from build123d import *

# Parameters (mm, degrees)
IZIM1_R                     = 3.5
IZIM1_R_2                   = 1.05
Y_KSEKLIK_EKSTR_ZYON1_DEPTH = 4
IZIM1_5_R                   = 0.5
Y_KSEKLIK_EKSTR_ZYON2_DEPTH = 1.8
IZIM2_R                     = 2.5
KES_EKSTR_ZYON1_DEPTH       = 2


with BuildPart() as part:
    # izim1 → Y_kseklik-Ekstr_zyon1 (new body)
    with BuildSketch(Plane(origin=(0, 0, 0), x_dir=(0, 0, -1), z_dir=(1, 0, 0))):
        with Locations((585.534826128, 415.055894204)):
            Circle(IZIM1_R)
        with Locations((585.534826128, 415.055894204)):
            Circle(IZIM1_R_2, mode=Mode.SUBTRACT)
    extrude(amount=Y_KSEKLIK_EKSTR_ZYON1_DEPTH)

    # izim1_5 → Y_kseklik-Ekstr_zyon2 (add)
    with BuildSketch(Plane(origin=(0, 0, 0), x_dir=(0, 0, -1), z_dir=(1, 0, 0))):
        with BuildLine():
            Line((583.367103568, 428.530198932), (582.052256525, 415.40476232))
            ThreePointArc((582.052256525, 415.40476232), (585.553599597, 418.555843854), (589.020937835, 415.367382833))
            Line((589.020937835, 415.367382833), (587.846970124, 428.506169262))
            ThreePointArc((587.846970124, 428.506169262), (585.617966971, 430.555894204), (583.367103568, 428.530198932))
        make_face()
        with Locations((585.566071769, 420.8810388)):
            Circle(IZIM1_5_R, mode=Mode.SUBTRACT)
        with Locations((585.57894519, 423.2810388)):
            Circle(IZIM1_5_R, mode=Mode.SUBTRACT)
        with Locations((585.591818611, 425.6810388)):
            Circle(IZIM1_5_R, mode=Mode.SUBTRACT)
        with Locations((585.604692031, 428.0810388)):
            Circle(IZIM1_5_R, mode=Mode.SUBTRACT)
    extrude(amount=Y_KSEKLIK_EKSTR_ZYON2_DEPTH)

    # izim2 → Kes-Ekstr_zyon1 (cut)
    with BuildSketch(Plane(origin=(4, 0, 0), x_dir=(0, 0, -1), z_dir=(1, 0, 0))):
        with Locations((585.534826128, 415.055894204)):
            Circle(IZIM2_R)
    extrude(amount=-KES_EKSTR_ZYON1_DEPTH, mode=Mode.SUBTRACT)


solid = part.part
Work out the finished part from the listing and answer in its coordinate system (mm). A direction names the side the tool comes from. Give positions to 0.01 mm unless a question says otherwise; leave off trailing zeros. Order: outer loops, then holes, each group sorted by start corner. A loop starts at its lowest first (then second) coordinate and runs counter-clockwise, first axis right, second up. Notation, with made-up numbers: (22.25, -25.75) - (66.25, -25.75) arc R23 ccw to (66.25, 7.25) - close; hole circle Ø3 at (26, 21). An arc over 180 degrees is marked (long way). Answer as CSV lines item,"result". Start each with the question number.
Q1. Find the intervals of material crossed by L1, parallel to Y at x = 2.6, z = -585.5; L2, parallel to X at y = 418.5, z = -584.25; L3, parallel to Z at x = 3.25, y = 417, in increasing order. Write a range as [from, to].
Q2. The part is cut by section D-D (x = 2.55). Write down the section's boundary in (y, z).
Q3. For faces 4 (the face through (2, 415, -587)), 5 (the face through (0.887, 430.555, -585.664)), determine the directions among +Z, -Z, +X, -X, +Y, -Y from which every point of the face is accessible in a straight line to the end or side of a thin tool.
Q4. The part is cut by section A-A (y = 417.75). Write down the section's boundary in (x, z).
Q5. The mould has two halves that part along Y. Classify faces 1 (the face through (0.887, 421.845, -588.442)), 2 (the face through (1.8, 423.1, -586.3)), 3 (the face through (0.89, 420.44, -585.8)): +Y half, -Y half, draft (parallel to the pull), parting line (faces both ways), or undercut.
Q6. The part is cut by section C-C (x = 0.45). Write down the section's boundary in (y, z), then the cut area to 3 significant figures.
Q7. The part is cut by section B-B (z = -584). Write down the section's boundary in (x, y), then the cut area to 3 significant figures.
Q8. Given pin 1 Ø1.3 at (y, z) = (415.06, -585.53) entering from -X; pin 2 Ø2 at (y, z) = (419.5, -583.5) entering from +X; pin 3 Ø1.5 at (x, z) = (3, -583.5) entering from +Y; pin 4 Ø1.5 at (x, y) = (1, 421.5) entering from +Z, each flat-ended and moving along its own axis, determine where each tip first touches the part or whether it passes through.
Check result:
1,L1,"y = [411.56, 412.56], [417.56, 418.56]"
1,L2,"x = [0, 1.8]"
1,L3,"z = [-588.45, -587.11], [-583.96, -582.62]"
2,outline,"circle Ø7 at (415.06, -585.53); hole circle Ø5 at (415.06, -585.53)"
3,face 4,"+X"
3,face 5,"+X, -X, +Y"
4,outline,"(0, -588.81) - (1.8, -588.81) - (1.8, -587.77) - (4, -587.77) - (4, -583.3) - (1.8, -583.3) - (1.8, -582.29) - (0, -582.29) - close"
5,face 1,"+Y half"
5,face 2,"draft"
5,face 3,"undercut"
6,outline,"(415.37, -589.02) - (428.51, -587.85) arc R2.25 ccw to (428.53, -583.37) - (415.4, -582.05) arc R3.5 ccw (long way) to start; hole circle Ø2.1 at (415.06, -585.53); hole circle Ø1 at (420.88, -585.57); hole circle Ø1 at (423.28, -585.58); hole circle Ø1 at (425.68, -585.59); hole circle Ø1 at (428.08, -585.6)"
6,area,"97.1 mm²"
7,outline,"(0, 411.91) - (4, 411.91) - (4, 413.08) - (2, 413.08) - (2, 417.03) - (4, 417.03) - (4, 418.2) - (1.8, 418.2) - (1.8, 429.88) - (0, 429.88) - close"
7,area,"38.3 mm²"
8,pin 1,"passes through"
8,pin 2,"stops at x = 1.8"
8,pin 3,"stops at y = 418.31"
8,pin 4,"stops at z = -582.59"
